Autodesk Inventor part; units mm, degrees
ref_plane "Work Plane1" through (0, 12.7, 0) normal (0, 1, 0) x (-1, 0, 0)
ref_plane "YZ Plane" through (0, 0, 0) normal (1, 0, 0) x (0, 1, 0)
ref_plane "XY Plane" through (0, 0, 0) normal (0, 0, 1) x (1, 0, 0)
sketch "Sketch1" plane through (0, 0, 0) normal (0, 0, 1) x (1, 0, 0)
  circle A0 centre (0, 0) radius 12.7
  dimension "d0" = 25.4
extrude "Extrusion1" add sketch "Sketch1" against normal blind 11.1252
sketch "Sketch2" plane through (0, 0, 0) normal (0, 0, 1) x (1, 0, 0)
  circle A0 centre (0, 0) radius 12.7
  circle A1 centre (0, 0) radius 6.35
  dimension "d3" = 12.7
extrude "Extrusion2" cut sketch "Sketch2" against normal up to next contours A1
chamfer "Chamfer1" distance 0.3969 angle 45 4 edges at (-12.7, 0, 0) (-12.7, 0, -11.1252) (-6.35, 0, 0) (-6.35, 0, -11.1252)
ref_plane "Work Plane1" through (0, 12.7, 0) normal (0, 1, 0) x (-1, 0, 0)
sketch "Sketch3" plane through (0, 12.7, 0) normal (0, 1, 0) x (-1, 0, 0)
  line L0 (12.3031, -11.1252) -> (-12.3031, -11.1252)
  line L1 (12.7, -0.3969) -> (12.7, -10.7283)
  point P0 (0, 0)
  point P1 (0, -5.5626)
  point P2 (0, -11.1252)
  point P3 (12.7, -5.5626)
hole "Hole1" at (0, 12.7, -5.5626) direction (0, -1, 0) diameter 4.9784 end up to surface
properties part number "SC-8-F"
Design review of the part built by this model. Coordinates are the model's own, in mm. A direction names the side the tool comes from. Coordinates: 2 decimals unless noted, no trailing zeros. Order: outer loops, then holes, each group sorted by start corner. A loop starts at its lowest first (then second) coordinate and runs counter-clockwise, first axis right, second up. Notation, with made-up numbers: (31.25, -26) - (86.25, -26) arc R16 ccw to (86.25, 2) - close; hole circle Ø2 at (0.5, -6.75). An arc over 180 degrees is marked (long way). Answer in a Markdown table with one row per item.
(1) Consider section A-A on x = 0. State the section outline as (y, z) points, plus the area to 3 significant figures.
Checked values:
| item | result |
|---|---|
| outline | (-12.7, -10.73) - (-12.3, -11.13) - (-6.75, -11.13) - (-6.35, -10.73) - (-6.35, -0.4) - (-6.75, 0) - (-12.3, 0) - (-12.7, -0.4) - close; (6.35, -10.73) - (6.75, -11.13) - (12.3, -11.13) - (12.7, -10.73) - (12.7, -8.05) - (6.35, -8.05) - close; (6.35, -3.07) - (12.7, -3.07) - (12.7, -0.4) - (12.3, 0) - (6.75, 0) - (6.35, -0.4) - close |
| area | 109 mm^2 |
(2) Wall thickness on line 1 along Y through (x, z) = (0, -8.5); line 2 along Z through (x, y) = (0, 8.25); line 3 along X through (y, z) = (2.5, -2.5): over which ranges is each line inside the solid? List them lowest first. Write a range as from..to.
Checked values:
| item | result |
|---|---|
| line 1 | -12.7..-6.35, 6.35..12.7 |
| line 2 | -11.13..-8.05, -3.07..0 |
| line 3 | -12.45..-5.84, 5.84..12.45 |
(3) The part is to be moulded in two halves that separate along Y. For faces 3 (the cylindrical face through (-2.75, -12.4, -5.49)), 4 (the flat face through (5, -5, 0)), 5 (the cylindrical face through (-1.38, -6.2, -5.49)), say which applies: released by +Y, released by -Y, zero draft, split by the parting line, or undercut.
Checked values:
| item | result |
|---|---|
| face 3 | split by the parting line |
| face 4 | zero draft |
| face 5 | undercut |
(4) Consider section C-C on z = -10. State the section outline as (x, y) points.
Checked values:
| item | result |
|---|---|
| outline | circle Ø25.4 at (0, 0); hole circle Ø12.7 at (0, 0) |
(5) Consider section B-B on y = 0. State the section outline as (x, z) points.
Checked values:
| item | result |
|---|---|
| outline | (-12.7, -10.73) - (-12.3, -11.13) - (-6.75, -11.13) - (-6.35, -10.73) - (-6.35, -0.4) - (-6.75, 0) - (-12.3, 0) - (-12.7, -0.4) - close; (6.35, -10.73) - (6.75, -11.13) - (12.3, -11.13) - (12.7, -10.73) - (12.7, -0.4) - (12.3, 0) - (6.75, 0) - (6.35, -0.4) - close |
(6) Clearance check with flat-ended pins moving along their axes: pin 1 (8 mm diameter, centred on x = -1, y = 7.5, fed in from +Z); pin 2 (3 mm diameter, centred on x = 2, z = -1.5, fed in from -Y); pin 3 (1 mm diameter, centred on y = 6.5, z = -7.5, fed in from -X). State where each tip first meets the part, or that it passes through.
Checked values:
| item | result |
|---|---|
| pin 1 | z = 0 |
| pin 2 | y = -12.69 |
| pin 3 | x = -11.19 |
(7) For faces 1 (the flat face through (5, -5, -11.125)), 2 (the cylindrical face through (-0.11, 9.22, -8.05)), list the 3-axis set-ups (+Z, -Z, +X, -X, +Y, -Y) from which the entire face can be reached by the end or side of a thin tool; tool diameter is ignored.
Checked values:
| item | result |
|---|---|
| face 1 | -Z, +X, -X, +Y, -Y |
| face 2 | +Y |
(8) Consider section D-D on z = -6.5. State the section outline as (x, y) points.
Checked values:
| item | result |
|---|---|
| outline | (-2.31, 5.92) - (-2.31, 12.49) arc R12.7 ccw (long way) to (2.31, 12.49) - (2.31, 5.92) arc R6.35 cw (long way) to start |
